The listing builds one solid part. Answer for the finished solid, in the listing's coordinates (mm). A direction names the side the tool comes from. Coordinates: 2 decimals unless noted, no trailing zeros. Order: outer loops, then holes, each group sorted by start corner. A loop starts at its lowest first (then second) coordinate and runs counter-clockwise, first axis right, second up. Notation, with made-up numbers: (75, 13) -> (134, 13) arc R25 cw to (134, 38) -> close; hole circle Ø5 at (87, 12). An arc over 180 degrees is marked (long way). Put each result on its own line as item: value. Start each with the question number.
```python
from build123d import *

# Parameters (mm, degrees)
F1_DEPTH  = 5
F3_DEPTH  = 15
F8_DEPTH  = 2.5
F9_W      = 78
F9_H      = 55.5
F9_R      = 2
F10_DEPTH = 25
F11_R     = 11.15
F11_R_2   = 2.65
F12_DEPTH = 25
F13_R     = 8.15
F14_DEPTH = 25
F16_DEPTH = 25
F17_W     = 10
F17_H     = 5
F17_R     = 2.5


with BuildPart() as f1:
    # F0 (on Top) → F1 (new body)
    with BuildSketch(Plane.XY):
        with BuildLine():
            Line((20.3815252042, 117.1415335559), (0, 0))
            Line((0, 0), (487.8028212909, 0))
            Line((487.8028212909, 0), (467.4212960867, 117.1415335559))
            ThreePointArc((467.4212960867, 117.1415335559), (433.2669551721, 176.5315404118), (368.9014106455, 200))
            Line((368.9014106455, 200), (118.9014106455, 200))
            ThreePointArc((118.9014106455, 200), (54.5358661189, 176.5315404118), (20.3815252042, 117.1415335559))
        make_face()
    extrude(amount=-F1_DEPTH)

    # F2 (on face) → F3 (join)
    with BuildSketch(Plane.XY):
        with BuildLine():
            Line((368.9014106455, 200), (118.9014106455, 200))
            ThreePointArc((118.9014106455, 200), (54.5358661189, 176.5315404118), (20.3815252042, 117.1415335559))
            Line((20.3815252042, 117.1415335559), (35.3815252042, 117.1415335559))
            ThreePointArc((35.3815252042, 117.1415335559), (65.0954102081, 165.8969986874), (118.9014106455, 185))
            Line((118.9014106455, 185), (368.9014106455, 185))
            ThreePointArc((368.9014106455, 185), (422.7074110828, 165.8969986874), (452.4212960867, 117.1415335559))
            Line((452.4212960867, 117.1415335559), (467.4212960867, 117.1415335559))
            ThreePointArc((467.4212960867, 117.1415335559), (433.2669551721, 176.5315404118), (368.9014106455, 200))
        make_face()
    extrude(amount=F3_DEPTH)

    # F6: sweep along a path in F5
    with BuildLine(Plane.XY.offset(15)) as f6_path:
        ThreePointArc((20.3815252042, 117.1415335559), (54.5358661189, 176.5315404118), (118.9014106455, 200))
        Line((118.9014106455, 200), (368.9014106455, 200))
        ThreePointArc((368.9014106455, 200), (433.2669551721, 176.5315404118), (467.4212960867, 117.1415335559))
    # F4 (on face) → F6 (sweep, cut)
    with BuildSketch(Plane.XZ.offset(-117.1415335559)):
        with BuildLine():
            ThreePointArc((20.3815252042, 2.5), (29.2203599691, 6.1611652352), (32.8815252042, 15))
            Line((32.8815252042, 15), (20.3815252042, 15))
            Line((20.3815252042, 15), (20.3815252042, 2.5))
        make_face()
    sweep(path=f6_path.line, mode=Mode.SUBTRACT)

    # F7 (on face) → F8 (join)
    with BuildSketch(Plane.XY):
        Polygon((-15, 0), (0, 0), (20.3815252042, 117.1415335559), (5.3815252042, 117.1415335559), align=None)
        Polygon((0, 0), (15, 0), (35.3815252042, 117.1415335559), (20.3815252042, 117.1415335559), align=None)
        Polygon((452.4212960867, 117.1415335559), (473.0281739523, 0), (487.8028212909, 0), (467.4212960867, 117.1415335559), align=None)
        Polygon((467.4212960867, 117.1415335559), (487.8028212909, 0), (503.0281739523, 0), (482.4212960867, 117.1415335559), align=None)
    extrude(amount=F8_DEPTH)

    # F9 (on face) → F10 (cut)
    with BuildSketch(Plane(origin=(0, 0, -5), x_dir=(1, 0, 0), z_dir=(0, 0, -1))):
        with Locations((242.9, -120.25)):
            Rectangle(F9_W, F9_H)
        with Locations((200.2686832967, -149.75)):
            Circle(F9_R)
        with Locations((200.2686832967, -90.75)):
            Circle(F9_R)
        with Locations((285.2686832967, -90.75)):
            Circle(F9_R)
        with Locations((285.2686832967, -149.75)):
            Circle(F9_R)
    extrude(amount=-F10_DEPTH, mode=Mode.SUBTRACT)

    # F11 (on face) → F12 (cut)
    with BuildSketch(Plane(origin=(0, 0, -5), x_dir=(1, 0, 0), z_dir=(0, 0, -1))):
        Polygon((391.9, -78.9489291724), (399.65, -74.4744645862), (399.65, -65.5255354138), (391.9, -61.0510708276), (384.15, -65.5255354138), (384.15, -74.4744645862), align=None)
        with Locations((361.9, -70)):
            Circle(F11_R)
        with Locations((361.9, -100)):
            Circle(F11_R_2)
        with Locations((391.9, -100)):
            Circle(F11_R_2)
    extrude(amount=-F12_DEPTH, mode=Mode.SUBTRACT)

    # F13 (on face) → F14 (cut)
    with BuildSketch(Plane.XY):
        with Locations((100, 70)):
            Circle(F13_R)
    extrude(amount=-F14_DEPTH, mode=Mode.SUBTRACT)

    # F15 (on face) → F16 (join)
    with BuildSketch(Plane.XY):
        Polygon((40.456642758, 117.1415335559), (32.2544592526, 70), (62.2544592526, 70), (70.456642758, 117.1415335559), align=None)
        Polygon((415.343357242, 117.1415335559), (423.5455407474, 70), (453.5455407474, 70), (445.343357242, 117.1415335559), align=None)
    extrude(amount=F16_DEPTH)

    # F19: sweep along a path in F18
    with BuildLine(Plane.XY) as f19_path:
        ThreePointArc((55.456642758, 117.1415335559), (77.6120171917, 155.0538221629), (118.9014106455, 170))
        Line((118.9014106455, 170), (368.9014106455, 170))
        ThreePointArc((368.9014106455, 170), (409.4264963221, 154.9669307173), (430.343357242, 117.1415335559))
        Line((430.343357242, 117.1415335559), (431.8368507266, 107.2536886334))
    # F17 (on face) → F19 (sweep)
    with BuildSketch(Plane(origin=(0, 117.1415335559, 0), x_dir=(-1, 0, 0), z_dir=(0, 1, 0))):
        with Locations((-55.456642758, 2.5)):
            Rectangle(F17_W, F17_H)
        with Locations((-55.456642758, -4)):
            Circle(F17_R)
    sweep(path=f19_path.line)


solid = f1.part
```
(1) Find the intervals of material crossed by L1, parallel to Y at x = 361, z = -1; L2, parallel to Y at x = 232.5, z = 1; L3, parallel to X at y = 149.75, z = -3.1, in increasing order.
(2) A tool of negligible diameter and unlimited length cuts with its end or side. For faces 4 (the flat face through (477.755, 57.751, -2.465)), 5 (the flat face through (2, 59, 0)), 6 (the cylindrical face through (411.436, 159.709, 2.535)), from which of +Z, -Z, +X, -X, +Y, -Y can it reach the whole face along a straight path? Write none if from no direction.
(3) Each of these flat-tipped pins is pushed along its axis until it touches: P1, Ø20, axis at x = 361.9, y = 70, coming from the -Z side; P2, Ø4.5, axis at x = 285.27, y = 149.75, coming from the +Z side; P3, Ø10, axis at x = 29.5, z = 7.5, coming from the -Y side; P4, Ø4, axis at y = 113, z = -3, coming from the -X side. Where does it stop, or does it pass through?
(4) The part is cut by section A-A on y = 24. Determine the outline of the cut face in (x, z).
(5) For a pull along Y with two mould halves and no side action, classify faces 1 (the flat face through (242, 185, 7)), 2 (the cylindrical face through (55.29, 177.16, -1.3)), 3 (the flat face through (47, 70, 12)) as released by +Y, released by -Y, zero draft, split by the parting line, or undercut.
Worked out:
1. L1: 0 to 58.89, 81.11 to 97.51, 102.49 to 200
1. L2: 165.08 to 174.92, 185 to 200
1. L3: 32.16 to 198.27, 202.27 to 283.27, 287.27 to 455.65
2. face 4: -Z, +X, +Y
2. face 5: -Z, -X, +Y
2. face 6: +Z
3. P1: through
3. P2: z = 0
3. P3: y = 70
3. P4: x = 19.31
4. outline: (-10.82, 0) -> (4.18, 0) -> (4.18, -5) -> (483.63, -5) -> (483.63, 0) -> (498.81, 0) -> (498.81, 2.5) -> (468.81, 2.5) -> (468.81, 0) -> (19.18, 0) -> (19.18, 2.5) -> (-10.82, 2.5) -> close
5. face 1: undercut
5. face 2: released by +Y
5. face 3: released by -Y
